Read the model definition and answer for the solid it produces. Units are mm, in the model's axes. Face numbers are marked on the shaded views. A direction names the side the tool comes from. Give positions to 0.01 mm unless a question says otherwise; leave off trailing zeros. Write each loop counter-clockwise with the first axis right and the second up, starting at its lowest first coordinate (ties: lowest second). Pieces come first, ordered by that corner, then holes. Notation, with made-up numbers: (-37, 43.25) -> (1, 43.25) arc R22 ccw to (1, 81.25) -> close; hole circle Ø7 at (-10, -24). An arc over 180 degrees is marked (long way). Answer as CSV lines item,"result". Start each with the question number.
1. The part is cut by section D-D, the plane z = 2.25. Determine the outline of the cut face in (x, y).
2. Find the intervals of material crossed by line 1 (X direction, y = 1, z = 0); line 2 (X direction, y = -3.5, z = 3.5); line 3 (X direction, y = -4.25, z = -0.75), in increasing order.
3. A tool of negligible diameter and unlimited length cuts with its end or side. For the marked faces 1 and 2, from which of +Z, -Z, +X, -X, +Y, -Y can it reach the whole face along a straight path? Write none if from no direction.
4. The part is cut by section C-C, the plane x = 28.2. Determine the outline of the cut face in (y, z), and give its area (3 significant figures).
5. The part is cut by section B-B, the plane z = 0. Determine the outline of the cut face in (x, y).
6. The part is cut by section A-A, the plane y = 0. Determine the outline of the cut face in (x, z), and give its area (3 significant figures).
7. Given pin 1 (1 mm diameter, centred on x = 18, y = 0.5, fed in from +Z); pin 2 (1.5 mm diameter, centred on y = 1, z = 1, fed in from -X); pin 3 (1.1 mm diameter, centred on x = 28.2, z = 0, fed in from -Y), each flat-ended and moving along its own axis, determine where each tip first touches the part or whether it passes through.
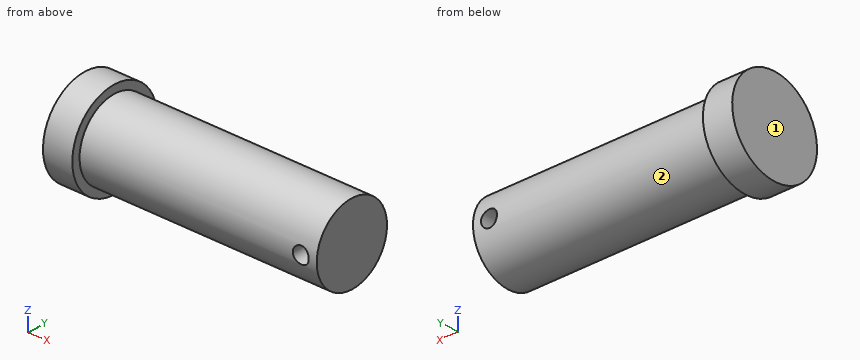
from build123d import *

# Parameters (mm, degrees)
SKETCH1_R               = 2.9
BOSS_EXTRUDE1_DEPTH     = 20
CUT_EXTRUDE1_DEPTH      = 10
CUT_EXTRUDE1_DEPTH_BACK = 10
SKETCH2_R               = 0.6
SKETCH3_R               = 3.5
BOSS_EXTRUDE2_DEPTH     = 2.2
SCALE1_SCALE            = 1.5


with BuildPart() as part:
    # Sketch1 → Boss-Extrude1 (new body)
    with BuildSketch(Plane(origin=(0, 0, 0), x_dir=(0, 0, -1), z_dir=(1, 0, 0))):
        Circle(SKETCH1_R)
    extrude(amount=BOSS_EXTRUDE1_DEPTH)

    # Sketch2 → Cut-Extrude1 (cut, two sides: drawn at the far end of the back side and taken through both)
    with BuildSketch(Plane(origin=(0, 0, 0), x_dir=(1, 0, 0), z_dir=(0, 1, 0)).offset(-CUT_EXTRUDE1_DEPTH_BACK)):
        with Locations(Location((18.8, 0, 0), (0, 0, 90))):
            Circle(SKETCH2_R)
    extrude(amount=CUT_EXTRUDE1_DEPTH + CUT_EXTRUDE1_DEPTH_BACK, mode=Mode.SUBTRACT)

    # Sketch3 → Boss-Extrude2 (add)
    with BuildSketch(Plane.ZY):
        Circle(SKETCH3_R)
    extrude(amount=-BOSS_EXTRUDE2_DEPTH)


with BuildPart() as part_1:
    # Scale1: scaled about (0, 0, 0)
    add(part.part.scale(SCALE1_SCALE))


solid = part_1.part
Results found:
1,outline,"(0, -4.74) -> (3.3, -4.74) -> (3.3, -3.72) -> (30, -3.72) -> (30, 3.72) -> (3.3, 3.72) -> (3.3, 4.74) -> (0, 4.74) -> close"
2,line 1,"x = 0 to 27.3, 29.1 to 30"
2,line 2,"x = 0 to 3.3"
2,line 3,"x = 0 to 27.7, 28.7 to 30"
3,face 1,"+Z, -Z, -X, +Y, -Y"
3,face 2,"+X"
4,outline,"(-4.26, -0.9) arc R4.35 ccw to (4.26, -0.9) -> close; (-4.26, 0.9) -> (4.26, 0.9) arc R4.35 ccw to start"
4,area,"43.9 mm²"
5,outline,"(0, -5.25) -> (3.3, -5.25) -> (3.3, -4.35) -> (27.3, -4.35) -> (27.3, 4.35) -> (3.3, 4.35) -> (3.3, 5.25) -> (0, 5.25) -> close; (29.1, -4.35) -> (30, -4.35) -> (30, 4.35) -> (29.1, 4.35) -> close"
6,outline,"(0, -5.25) -> (3.3, -5.25) -> (3.3, -4.35) -> (30, -4.35) -> (30, 4.35) -> (3.3, 4.35) -> (3.3, 5.25) -> (0, 5.25) -> close; hole circle Ø1.8 at (28.2, 0)"
6,area,"264 mm²"
7,pin 1,"stops at z = 4.35"
7,pin 2,"stops at x = 0"
7,pin 3,"passes through"
